CAD build for the part. Positions are in the model's coordinates, mm. A direction names the side the tool comes from. Coordinates: 2 decimals unless noted, no trailing zeros. Order: outer loops, then holes, each group sorted by start corner. A loop starts at its lowest first (then second) coordinate and runs counter-clockwise, first axis right, second up. Notation, with made-up numbers: M 78.25,67.25 L 108.25,67.25 A22 cw 108.25,83.25 Z; hole C 14.5,52.25 d8. An arc over 180 degrees is marked long. One line per item, written item: value.
from build123d import *

# Parameters (mm, degrees)
BOSS_EXTRUDE2_DEPTH = 13
SKETCH3_R           = 38.614889052
BOSS_EXTRUDE3_DEPTH = 44


with BuildPart() as part:
    # Sketch1 → Boss-Extrude2 (new body)
    with BuildSketch(Plane(origin=(0, 0, 0), x_dir=(1, 0, 0), z_dir=(0, 1, 0))):
        with BuildLine():
            Line((132.11743751, -48.51341168), (94.01743751, -70.510456937))
            ThreePointArc((94.01743751, -70.510456937), (84.828443129, -74.316663034), (74.96743751, -75.614889052))
            Line((74.96743751, -75.614889052), (17.81743751, -75.614889052))
            ThreePointArc((17.81743751, -75.614889052), (11.548173881, -74.952515636), (5.555749824, -72.994644622))
            Line((5.555749824, -72.994644622), (-60.707020947, -43.319675524))
            ThreePointArc((-60.707020947, -43.319675524), (-69.317811507, -35.941035728), (-72.53256249, -25.066505144))
            Line((-72.53256249, -25.066505144), (-72.53256249, 65.185110948))
            ThreePointArc((-72.53256249, 65.185110948), (-69.603630301, 72.256178759), (-62.53256249, 75.185110948))
            Line((-62.53256249, 75.185110948), (128.46743751, 75.185110948))
            ThreePointArc((128.46743751, 75.185110948), (135.538505322, 72.256178759), (138.46743751, 65.185110948))
            Line((138.46743751, 65.185110948), (138.46743751, -37.514889052))
            ThreePointArc((138.46743751, -37.514889052), (136.765960139, -43.864889052), (132.11743751, -48.51341168))
        make_face()
    extrude(amount=BOSS_EXTRUDE2_DEPTH)

    # Sketch3 → Boss-Extrude3 (add)
    with BuildSketch(Plane(origin=(0, 0, 0), x_dir=(1, 0, 0), z_dir=(0, 1, 0))):
        with Locations((74.46743751, -37)):
            Circle(SKETCH3_R)
    extrude(amount=-BOSS_EXTRUDE3_DEPTH)


solid = part.part
Q1. Drill centre lines: line 1 along Y through (x, z) = (36.5, -55); line 2 along X through (y, z) = (-36, 8); line 3 along Z through (x, y) = (89, -28). Where is each one in solid material? Low to high.
Recorded:
line 1: y = 0 to 13
line 2: x = 48.97 to 99.96
line 3: z = 1.22 to 72.78
Q2. Slice it at B-B (x = 25). List the corners of the cut face in (y, z), plus the area to 3 significant figures.
Recorded:
outline: M 0,-75.19 L 13,-75.19 L 13,75.61 L 0,75.61 Z
area: 1,960 mm^2
Q3. Pin check, flat tips, straight feed: pin 1 Ø3 at (x, y) = (46, -7) entering from -Z; pin 2 Ø1.5 at (x, z) = (-16.5, -47.5) entering from -Y. Stop position of each tip, or through.
Recorded:
pin 1: stops at z = 9.36
pin 2: stops at y = 0
Q4. Which spindle directions (+Z, -Z, +X, -X, +Y, -Y) get a long thin tool onto all of the face, cutting with end or side? Do faces 1 (the face through (35.89, -21.69, 35.3)), 2 (the face through (-27.112, 6.409, 58.365)). Say none if no direction does.
Recorded:
face 1: -Y
face 2: +Z, -X, +Y, -Y
Q5. Slice it at C-C (y = -9). List the corners of the cut face in (x, z), plus the area to 3 significant figures.
Recorded:
outline: C 74.47,37 d77.23
area: 4,680 mm^2
Q6. Slice it at A-A (z = -26.5). List the corners of the cut face in (x, y).
Recorded:
outline: M -72.53,0 L 138.47,0 L 138.47,13 L -72.53,13 Z
